Work out the finished part from the listing and answer in its coordinate system (mm). A direction names the side the tool comes from. Give positions to 0.01 mm unless a question says otherwise; leave off trailing zeros. Loops run counter-clockwise (first coordinate to the right, second up) from the corner with the lowest first, then second, coordinate; pieces in that order, holes last. Notation, with made-up numbers: M -11,40.25 L 40,40.25 A14 cw 40,53.25 Z; hole C -36,33 d10. An arc over 180 degrees is marked long. Write item = value, one per line. Start each with the question number.
1. Flat-ended cylindrical pins translate along their axes: pin 1 Ø5 at (x, z) = (-4.5, 13) entering from -Y; pin 2 Ø10 at (x, z) = (-30, 17.5) entering from +Y; pin 3 Ø1.5 at (x, z) = (-22, 5.5) entering from +Y. Find the tip coordinate at first contact, or state that the pin passes through.
2. The mould has two halves that part along Y. Classify faces 3 (the face through (1.398, -6.297, 9.86)), 4 (the face through (8, 1, 0)), 5 (the face through (27.715, -21.251, 13.079)): released by +Y, released by -Y, zero draft, split by the parting line, or undercut.
3. For faces 1 (the face through (-30.235, 23.183, 3.131)), 2 (the face through (17, -31, 6.35)), determine the directions among +Z, -Z, +X, -X, +Y, -Y from which every point of the face is accessible in a straight line to the end or side of a thin tool.
4. Section A-A on y = 0 is taken. Determine the outline of the cut face in (x, z) (3 decimals).
5. Section D-D on y = -9 is taken. Determine the outline of the cut face in (x, z).
6. Consider L1, parallel to Y at x = 0, z = 4.5; L2, parallel to X at y = 0, z = 12 (3 decimals). Determine where each line is inside the solid, lowest interval first. Write a range as [from, to].
7. Section C-C on z = 5.25 is taken. Determine the outline of the cut face in (x, y).
Autodesk Fusion 360 part; units mm, degrees
sketch "Roller_End_Cap_Outter" plane through (0, 0, 0) normal (0, 0, 1) x (1, 0, 0)
  circle A0 centre (0, 0) radius 38.1
  dimension "d2" = 76.2
extrude "Extrude1" add sketch "Roller_End_Cap_Outter" along normal blind 6.35
sketch "Roller_End_Cap_Inner" plane through (0, 0, 6.35) normal (0, 0, 1) x (-1, 0, 0)
  circle A0 centre (0, 0) radius 38.1
  circle A1 centre (0, 0) radius 34.925
  dimension "d7" = 69.85
extrude "Extrude3" add sketch "Roller_End_Cap_Inner" along normal blind 10 contours A1
sketch "Shaft Hole" plane through (0, 0, 16.35) normal (0, 0, 1) x (-1, 0, 0)
  circle A0 centre (0, 0) radius 34.925
  circle A1 centre (0, 0) radius 6.45
  dimension "d10" = 12.9
extrude "Extrude4" cut sketch "Shaft Hole" against normal through all contours A1
extrude "Extrude5" add 1 faces at (-25.3033, 1.7351, 16.35) along direction (0, 0, 1) blind 3.65
Verdict:
q1.pin_1 = -34.87
q1.pin_2 = 24.39
q1.pin_3 = 31.62
q2.face_3 = undercut
q2.face_4 = zero draft
q2.face_5 = split by the parting line
q3.face_1 = +Z, -Z
q3.face_2 = +Z
q4.outline = M -38.1,0 L -6.45,0 L -6.45,20 L -34.925,20 L -34.925,6.35 L -38.1,6.35 Z; M 6.45,0 L 38.1,0 L 38.1,6.35 L 34.925,6.35 L 34.925,20 L 6.45,20 Z
q5.outline = M -37.02,0 L 37.02,0 L 37.02,6.35 L 33.75,6.35 L 33.75,20 L -33.75,20 L -33.75,6.35 L -37.02,6.35 Z
q6.L1 = [-38.1, -6.45], [6.45, 38.1]
q6.L2 = [-34.925, -6.45], [6.45, 34.925]
q7.outline = C 0,0 d76.2; hole C 0,0 d12.9
